Model file for the job. Use its own axes, mm. Coordinates: 2 decimals unless noted, no trailing zeros. Write each loop counter-clockwise with the first axis right and the second up, starting at its lowest first coordinate (ties: lowest second). Pieces come first, ordered by that corner, then holes.
Q1. Pin check, flat tips, straight feed: P1, Ø6, axis at x = 100.5, z = 2, coming from the +Y side; P2, Ø1.5, axis at x = -39, z = 70, coming from the +Y side; P3, Ø4, axis at y = -84, z = -34.5, coming from the +X side. Stop position of each tip, or through.
Q2. Band-saw the part on B-B, the plane z = -64.5. Write the cut outline in (x, y).
Q3. Band-saw the part on A-A, the plane z = -6. Write the cut outline in (x, y).
Q4. Drill centre lines: probe 1 along Z at (x, y) = (32.5, 4); probe 2 along X at (y, z) = (-37, -98.5); probe 3 along Y at (x, z) = (-36, 41.5). Where is each one in solid material? Low to high.
Q5. Pull direction Y, two halves, no side cores. Call faces 1 (the flat face through (63.5, -31, -2)), 2 (the flat face through (-63.5, -25, -2)): released by +Y, released by -Y, zero draft, split by the parting line, or undercut.
from build123d import *

# Parameters (mm, degrees)
F0_W     = 127
F0_H     = 254
F1_DEPTH = 50.8
F2_R     = 38.1


with BuildPart() as f1:
    # F0 (on Front) → F1 (new body)
    with BuildSketch(Plane.XZ):
        Rectangle(F0_W, F0_H)
    extrude(amount=F1_DEPTH)

    # F2 (on face) → F3 (revolve)
    with BuildSketch(Plane.XZ.offset(50.8)):
        Circle(F2_R)
    revolve(axis=Axis((63.5, -50.8, 0), (0, 0, 1)))


solid = f1.part
Answer sheet:
1. P1: stops at y = 44.9
1. P2: stops at y = 0
1. P3: stops at x = 140.09
2. outline: (-63.5, -50.8) - (63.5, -50.8) - (63.5, 0) - (-63.5, 0) - close
3. outline: (-63.5, -50.8) - (-37.62, -50.8) arc R101.12 ccw (long way) to (-23.94, 0) - (-63.5, 0) - close; hole (37.62, -50.8) arc R25.88 ccw (long way) to (63.5, -24.92) - (63.5, -50.8) - close
4. probe 1: z = -38.1 to 38.1
4. probe 2: x = -63.5 to 63.5
4. probe 3: y = -50.8 to 0
5. face 1: undercut
5. face 2: zero draft
